```python
from build123d import *

# Parameters (mm, degrees)
F0_R      = 13.675
F1_DEPTH  = 6.7
F2_R      = 12.425
F3_DEPTH  = 5
F4_R      = 4.75
F5_DEPTH  = 0.2
F4_R_2    = 12.5
F4_R_3    = 9.5
F6_DEPTH  = 0.2
F8_DEPTH  = 6.701
F10_DEPTH = 6.701


with BuildPart() as f1:
    # F0 (on Front) → F1 (new body)
    with BuildSketch(Plane.XZ):
        Circle(F0_R)
    extrude(amount=F1_DEPTH)

    # F2 (on face) → F3 (cut)
    with BuildSketch(Plane.XZ.offset(6.7)):
        Circle(F2_R)
    extrude(amount=-F3_DEPTH, mode=Mode.SUBTRACT)

    # F4 (on face) → F5 (join)
    with BuildSketch(Plane(origin=(0, 0, 0), x_dir=(-1, 0, 0), z_dir=(0, 1, 0))):
        Circle(F4_R)
    extrude(amount=F5_DEPTH)

    # F4 (on face) → F6 (join)
    with BuildSketch(Plane(origin=(0, 0, 0), x_dir=(-1, 0, 0), z_dir=(0, 1, 0))):
        Circle(F4_R_2)
        Circle(F4_R_3, mode=Mode.SUBTRACT)
    extrude(amount=F6_DEPTH)

    # F7 (on face) → F8 (cut, through all)
    with BuildSketch(Plane(origin=(0, 0, 0), x_dir=(-1, 0, 0), z_dir=(0, 1, 0))):
        Polygon((-4.75, -2.175), (-4.75, 0), (-4.75, 2.175), (-5.75, 2.175), (-5.75, -2.175), align=None)
        Polygon((5.75, 2.175), (4.75, 2.175), (4.75, 0), (4.75, -2.175), (5.75, -2.175), align=None)
    extrude(amount=-F8_DEPTH, mode=Mode.SUBTRACT)

    # F9 (on face) → F10 (cut, through all)
    with BuildSketch(Plane(origin=(0, 0, 0), x_dir=(-1, 0, 0), z_dir=(0, 1, 0))):
        with BuildLine():
            Line((-2.175, -8.5), (-2.175, -9.2476686251))
            ThreePointArc((-2.175, -9.2476686251), (-1.0947940586, -9.4367063094), (0, -9.5))
            ThreePointArc((0, -9.5), (1.0947940586, -9.4367063094), (2.175, -9.2476686251))
            Line((2.175, -9.2476686251), (2.175, -8.5))
            Line((2.175, -8.5), (-2.175, -8.5))
        make_face()
        with BuildLine():
            ThreePointArc((2.175, 9.2476686251), (1.0947940586, 9.4367063094), (0, 9.5))
            ThreePointArc((0, 9.5), (-1.0947940586, 9.4367063094), (-2.175, 9.2476686251))
            Line((-2.175, 9.2476686251), (-2.175, 8.5))
            Line((-2.175, 8.5), (2.175, 8.5))
            Line((2.175, 8.5), (2.175, 9.2476686251))
        make_face()
    extrude(amount=-F10_DEPTH, mode=Mode.SUBTRACT)


solid = f1.part
```
CAD build for the part. Positions are in the model's coordinates, mm. A direction names the side the tool comes from. Round coordinates to 2 decimals unless told otherwise and drop trailing zeros. Loops run counter-clockwise (first coordinate to the right, second up) from the corner with the lowest first, then second, coordinate; pieces in that order, holes last. Notation, with made-up numbers: (40.25, 19.25) - (88.25, 19.25) arc R17 ccw to (88.25, 41.25) - close; hole circle Ø2 at (25, 89). An arc over 180 degrees is marked (long way). Return JSON: item names as keys, results as strings. Group by question number.
Q1. Tool access for faces 4 (the face through (5, -1, -2.175)), 5 (the face through (12.1, 0, -4)), 6 (the face through (-2.7, 0.2, 9.3)): list every direction of +Z, -Z, +X, -X, +Y, -Y with a clear straight run to the whole face (end or side of a thin tool).
Q2. Drill centre lines: line 1 along Z through (x, y) = (-0.25, -0.5); line 2 along Z through (x, y) = (0, -4.8) (3 decimals); line 3 along X through (y, z) = (-1.25, -0.5). Where is each one in solid material? Low to high. Write a range as [from, to].
Q3. Band-saw the part on B-B on z = -7.5. Give the cut face in (x, y), plus the area to 3 significant figures.
Q4. Two-plate mould, pull along Z, no slides. Class faces 1 (the face through (-9.86, -4.24, -7.56)), 2 (the face through (0, 0.2, 0)), 3 (the face through (7.4, -3.3, 11.5)): +Z half, -Z half, draft (parallel to the pull), parting line (faces both ways), or undercut.
Q5. Flat gauge pins, fed straight in: pin 1 Ø1 at (x, y) = (4, -5.5) entering from +Z; pin 2 Ø0.5 at (x, y) = (5, -0.5) entering from +Z; pin 3 Ø1 at (y, z) = (-5.5, -8.5) entering from +X. Where does each tip first touch, or does it go through?
Q6. Band-saw the part on A-A on y = -0.5. Give the cut face in (x, z) (3 decimals).
Q7. Band-saw the part on D-D on y = -5.25. Give the cut face in (x, z) (3 decimals), plus the area to 3 significant figures.
Q8. Band-saw the part on C-C on x = 6.25. Give the cut face in (y, z), plus the area to 3 significant figures.
Solutions:
{
 "1": {"face 4": "+Y, -Y", "face 5": "+Y", "face 6": "+Z, -Z, +X, -X, +Y"},
 "2": {"line 1": "z = [-13.67, -9.5], [-8.5, 8.5], [9.5, 13.67]", "line 2": "z = [-13.675, -12.425], [12.425, 13.675]", "line 3": "x = [-13.67, -5.75], [-4.75, 4.75], [5.75, 13.67]"},
 "3": {"outline": "(-11.43, -6.7) - (-9.91, -6.7) - (-9.91, -1.7) - (9.91, -1.7) - (9.91, -6.7) - (11.43, -6.7) - (11.43, 0) - (10, 0) - (10, 0.2) - (5.83, 0.2) - (5.83, 0) - (-5.83, 0) - (-5.83, 0.2) - (-10, 0.2) - (-10, 0) - (-11.43, 0) - close", "area": "55.8 mm^2"},
 "4": {"face 1": "undercut", "face 2": "draft", "face 3": "parting line"},
 "5": {"pin 1": "stops at z = 13.22", "pin 2": "stops at z = 12.82", "pin 3": "stops at x = 11.09"},
 "6": {"outline": "circle Ø27.35 at (0, 0); hole (-5.75, -2.175) - (-4.75, -2.175) - (-4.75, 2.175) - (-5.75, 2.175) - close; hole (-2.175, -9.248) arc R9.5 ccw to (2.175, -9.248) - (2.175, -8.5) - (-2.175, -8.5) - close; hole (-2.175, 8.5) - (2.175, 8.5) - (2.175, 9.248) arc R9.5 ccw to (-2.175, 9.248) - close; hole (4.75, -2.175) - (5.75, -2.175) - (5.75, 2.175) - (4.75, 2.175) - close"},
 "7": {"outline": "circle Ø27.35 at (0, 0); hole circle Ø24.85 at (0, 0)", "area": "102 mm^2"},
 "8": {"outline": "(-6.7, -12.16) - (0, -12.16) - (0, -10.83) - (0.2, -10.83) - (0.2, -7.15) - (0, -7.15) - (0, 7.15) - (0.2, 7.15) - (0.2, 10.83) - (0, 10.83) - (0, 12.16) - (-6.7, 12.16) - (-6.7, 10.74) - (-1.7, 10.74) - (-1.7, -10.74) - (-6.7, -10.74) - close", "area": "57.1 mm^2"}
}
